Answer from the drawing. Dimensions are ordinates in mm from the lowest x, y and z of the part. Give positions to 0.01 mm unless a question says otherwise; leave off trailing zeros. Loops run counter-clockwise (first coordinate to the right, second up) from the corner with the lowest first, then second, coordinate; pieces in that order, holes last.
(1) Find section B-B, the plane x = 24.13. State how many separate pieces and enclosed holes the cut face has, then the cut area to 3 significant figures.
(2) Find section A-A, the plane y = 16.51. Write down the section's boundary in (x, z) (1 decimal).
(3) This flat-tipped pin is pushed along its axis until it touches: P1, Ø4, axis at x = 19.05, y = 146.05, coming from the -Z side. Where does it stop, or does it pass through?
(4) Straight lines are drawn through the part: probe 1 along X at (y, z) = (146.05, 1.25); probe 2 along Y at (x, z) = (36.5, 3.25); probe 3 along Y at (x, z) = (27, 0.45). For each, find the intervals that lie inside material, in ascending order.
(5) Find section D-D, the plane y = 146.05. Write down the section's boundary in (x, z).
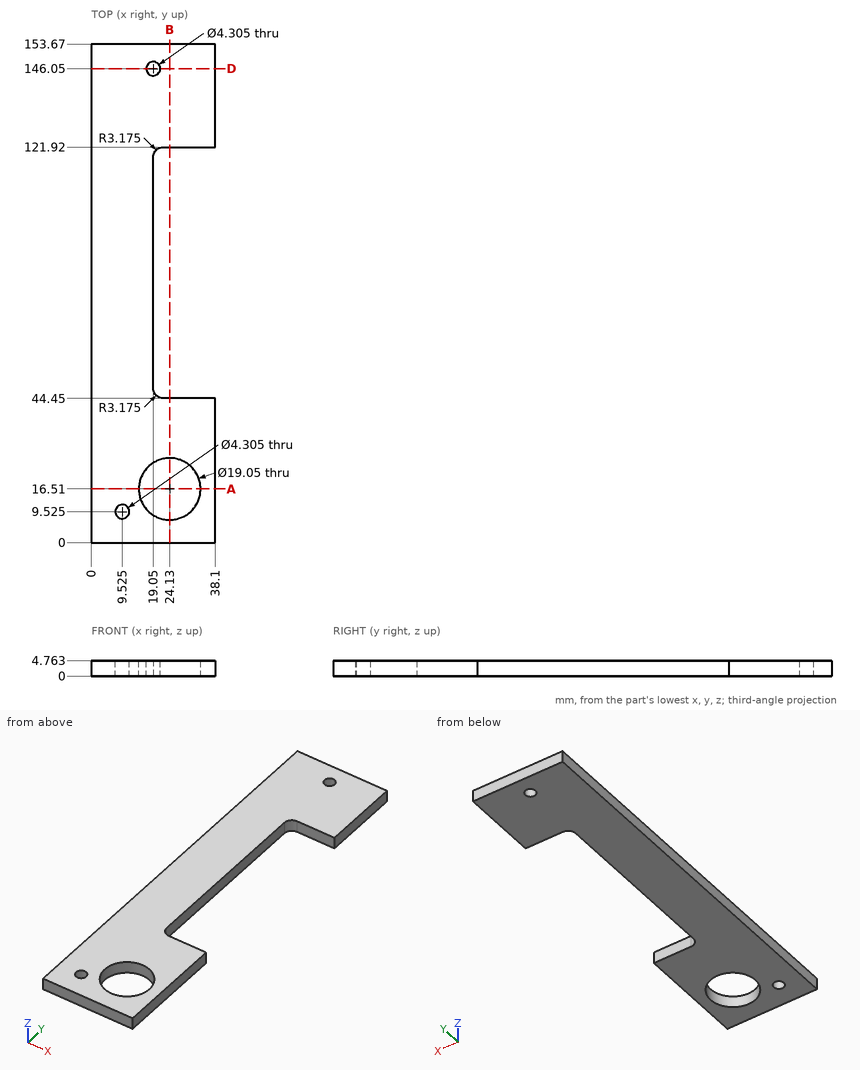
Entries:
1. separate pieces: 3
1. enclosed holes: 0
1. area: 272 mm2
2. outline: (0, 0) - (14.6, 0) - (14.6, 4.8) - (0, 4.8) - close; (33.7, 0) - (38.1, 0) - (38.1, 4.8) - (33.7, 4.8) - close
3. P1: passes through
4. probe 1: x = 0 to 16.9, 21.2 to 38.1
4. probe 2: y = 0 to 44.45, 121.92 to 153.67
4. probe 3: y = 0 to 7.43, 25.59 to 44.45, 121.92 to 153.67
5. outline: (0, 0) - (16.9, 0) - (16.9, 4.76) - (0, 4.76) - close; (21.2, 0) - (38.1, 0) - (38.1, 4.76) - (21.2, 4.76) - close
